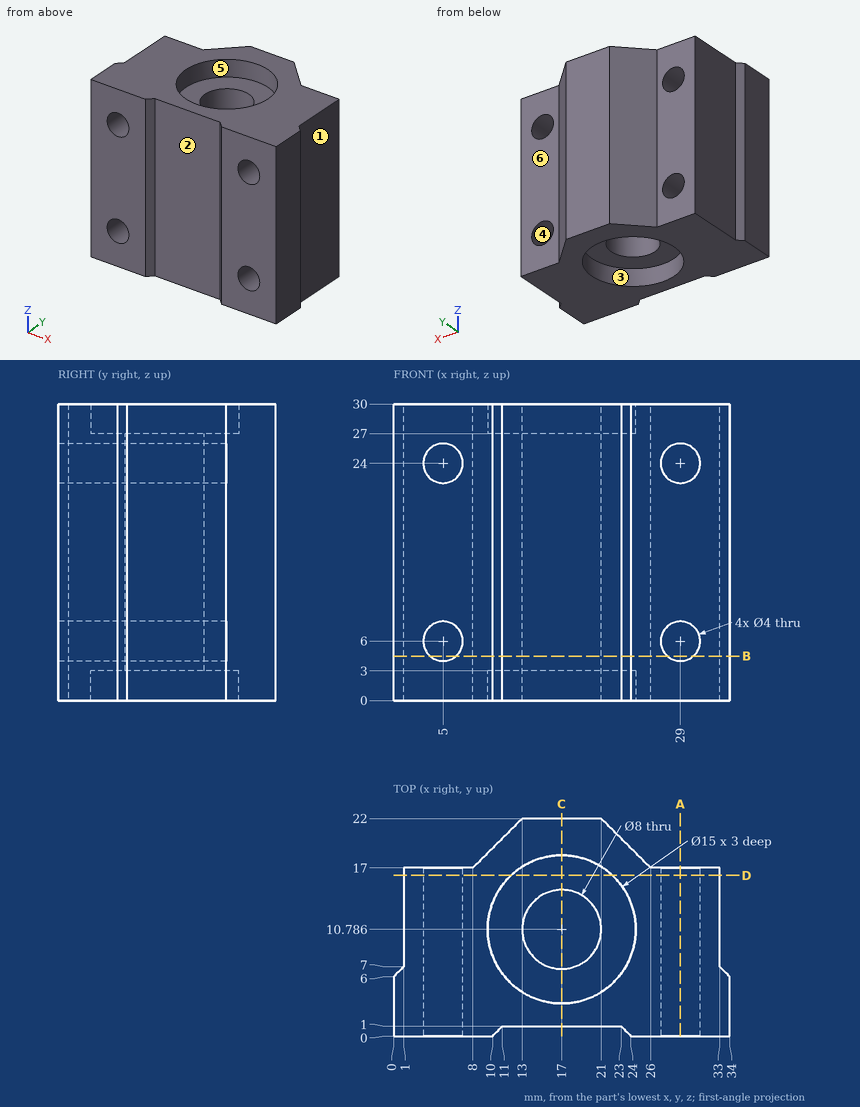
Print and shaded views of the part. All mm, measured from the part's lowest x, y and z. A direction names the side the tool comes from. Coordinates: 2 decimals unless noted, no trailing zeros. Order: outer loops, then holes, each group sorted by start corner. A loop starts at its lowest first (then second) coordinate and runs counter-clockwise, first axis right, second up.
(1) Tool access for the marked faces 1, 2 and 3: list every direction of +Z, -Z, +X, -X, +Y, -Y with a clear straight run to the whole face (end or side of a thin tool).
Check sheet entries:
face 1: +Z, -Z, +X, +Y
face 2: +Z, -Z, -Y
face 3: -Z
(2) Pin check, flat tips, straight feed: pin 1 Ø5 at (y, z) = (11.5, 6) entering from -X; pin 2 Ø3 at (x, z) = (29, 6) entering from -Y; pin 3 Ø4 at (x, z) = (28.5, 9.5) entering from +Y; pin 4 Ø5 at (y, z) = (10.5, 9) entering from +X. Stop position of each tip, or through.
Check sheet entries:
pin 1: stops at x = 1
pin 2: passes through
pin 3: stops at y = 17
pin 4: stops at x = 33
(3) Probe L1, parallel to Y at x = 17, z = 2.05; L2, parallel to X at y = 10.75, z = 28.5; L3, parallel to Z at x = 28.5, y = 8. List the from-to ranges inside material, lowest first.
Check sheet entries:
L1: y = 1 to 3.29, 18.29 to 22
L2: x = 1 to 9.5, 24.5 to 33
L3: z = 0 to 4.06, 7.94 to 22.06, 25.94 to 30
(4) Slice it at A-A, the plane x = 29. Write the cut outline in (y, z), and give its area (3 significant figures).
Check sheet entries:
outline: (0, 0) - (17, 0) - (17, 4) - (0, 4) - close; (0, 8) - (17, 8) - (17, 22) - (0, 22) - close; (0, 26) - (17, 26) - (17, 30) - (0, 30) - close
area: 374 mm2
(5) Pull direction Y, two halves, no side cores. Call the marked faces 4, 5 and 6: pulls with the +Y half, pulls with the -Y half, needs draft (parallel to the pull), parting line crosses it, or undercut.
Check sheet entries:
face 4: needs draft
face 5: undercut
face 6: pulls with the +Y half
(6) Slice it at C-C, the plane x = 17. Write the cut outline in (y, z).
Check sheet entries:
outline: (1, 0) - (3.29, 0) - (3.29, 3) - (6.79, 3) - (6.79, 27) - (3.29, 27) - (3.29, 30) - (1, 30) - close; (14.79, 3) - (18.29, 3) - (18.29, 0) - (22, 0) - (22, 30) - (18.29, 30) - (18.29, 27) - (14.79, 27) - close
(7) Slice it at B-B, the plane z = 4.5. Write the cut outline in (x, y).
Check sheet entries:
outline: (0, 0) - (3.68, 0) - (3.68, 17) - (1, 17) - (1, 7) - (0, 6) - close; (6.32, 0) - (10, 0) - (11, 1) - (23, 1) - (24, 0) - (27.68, 0) - (27.68, 17) - (26, 17) - (21, 22) - (13, 22) - (8, 17) - (6.32, 17) - close; (30.32, 0) - (34, 0) - (34, 6) - (33, 7) - (33, 17) - (30.32, 17) - close; hole circle Ø8 at (17, 10.79)
(8) Slice it at D-D, the plane y = 16.25. Write the cut outline in (x, z).
Check sheet entries:
outline: (1, 0) - (11.86, 0) - (11.86, 3) - (22.14, 3) - (22.14, 0) - (33, 0) - (33, 30) - (22.14, 30) - (22.14, 27) - (11.86, 27) - (11.86, 30) - (1, 30) - close; hole circle Ø4 at (5, 6); hole circle Ø4 at (5, 24); hole circle Ø4 at (29, 6); hole circle Ø4 at (29, 24)
